Geometry check sheet. Reference: the model listing, model coordinates, mm. A direction names the side the tool comes from. Round coordinates to 2 decimals unless told otherwise and drop trailing zeros. Order: outer loops, then holes, each group sorted by start corner. A loop starts at its lowest first (then second) coordinate and runs counter-clockwise, first axis right, second up.
```python
from build123d import *

# Parameters (mm, degrees)
SKETCH3_W           = 120
SKETCH3_H           = 50
BOSS_EXTRUDE1_DEPTH = 5
SKETCH6_R           = 2
CUT_EXTRUDE1_DEPTH  = 5


with BuildPart() as part:
    # Sketch3 → Boss-Extrude1 (new body)
    with BuildSketch(Plane(origin=(0, 0, 0), x_dir=(1, 0, 0), z_dir=(0, 1, 0))):
        Rectangle(SKETCH3_W, SKETCH3_H)
    extrude(amount=BOSS_EXTRUDE1_DEPTH)

    # Sweep1: sweep along a path in Sketch4
    with BuildLine(Plane.XY) as sweep1_path:
        Line((-50, 5), (-50, 25))
        ThreePointArc((-50, 25), (-47.071067812, 32.071067812), (-40, 35))
        Line((-40, 35), (40, 35))
        ThreePointArc((40, 35), (47.071067812, 32.071067812), (50, 25))
        Line((50, 25), (50, 5))
    # Sketch5 → Sweep1 (sweep)
    with BuildSketch(Plane(origin=(0, 5, 0), x_dir=(1, 0, 0), z_dir=(0, 1, 0))):
        with BuildLine():
            Line((-43.257688432, 6), (-43.257688432, -6))
            ThreePointArc((-43.257688432, -6), (-48.257688432, -11), (-53.257688432, -6))
            Line((-53.257688432, -6), (-53.257688432, 6))
            ThreePointArc((-53.257688432, 6), (-48.257688432, 11), (-43.257688432, 6))
        make_face()
    sweep(path=sweep1_path.line)

    # Sketch6 → Cut-Extrude1 (cut)
    with BuildSketch(Plane(origin=(0, 5, 0), x_dir=(1, 0, 0), z_dir=(0, 1, 0))):
        with Locations(Location((-56, 21, 0), (0, 0, 270))):
            Circle(SKETCH6_R)
        with Locations(Location((-50, 21, 0), (0, 0, 270))):
            Circle(SKETCH6_R)
        with Locations(Location((-50, -21, 0), (0, 0, 90))):
            Circle(SKETCH6_R)
        with Locations(Location((-56, -21, 0), (0, 0, 90))):
            Circle(SKETCH6_R)
        with Locations(Location((56, -21, 0), (0, 0, 270))):
            Circle(SKETCH6_R)
        with Locations(Location((50, -21, 0), (0, 0, 270))):
            Circle(SKETCH6_R)
        with Locations(Location((50, 21, 0), (0, 0, 90))):
            Circle(SKETCH6_R)
        with Locations(Location((56, 21, 0), (0, 0, 90))):
            Circle(SKETCH6_R)
    extrude(amount=-CUT_EXTRUDE1_DEPTH, mode=Mode.SUBTRACT)


solid = part.part
```
(1) Set-up check for faces 4 (the flat face through (53.258, 15, 0)), 5 (the flat face through (-53.258, 15, 0)), 6 (the cylindrical face through (42.278, 27.329, -0.084)), 7 (the cylindrical face through (-48.15, 15.14, -11)), 8 (the cylindrical face through (48.37, 14.86, 11)): record each of +Z, -Z, +X, -X, +Y, -Y from which the full face is reachable in a straight line by a thin tool's end or side.
Returned:
face 4: +Z, -Z, +X, +Y
face 5: +Z, -Z, -X, +Y
face 6: +Z, -Z
face 7: -Z
face 8: +Z
(2) Material ranges on line 1 (X direction, y = 3, z = 21); line 2 (X direction, y = 16, z = 4); line 3 (Y direction, x = 28.5, z = 3), recorded low to high.
Returned:
line 1: x = -60 to -58, -54 to -52, -48 to 48, 52 to 54, 58 to 60
line 2: x = -53.26 to -43.26, 43.26 to 53.26
line 3: y = 0 to 5, 28.26 to 38.26
(3) Sectioned sample at C-C, the plane x = 56. Record the cut outline in (y, z), and give its area (3 significant figures).
Returned:
outline: (0, -25) - (5, -25) - (5, -23) - (0, -23) - close; (0, -19) - (5, -19) - (5, 19) - (0, 19) - close; (0, 23) - (5, 23) - (5, 25) - (0, 25) - close
area: 210 mm2
(4) Sectioned sample at B-B, the plane z = 21. Record the cut outline in (x, y).
Returned:
outline: (-60, 0) - (-58, 0) - (-58, 5) - (-60, 5) - close; (-54, 0) - (-52, 0) - (-52, 5) - (-54, 5) - close; (-48, 0) - (48, 0) - (48, 5) - (-48, 5) - close; (52, 0) - (54, 0) - (54, 5) - (52, 5) - close; (58, 0) - (60, 0) - (60, 5) - (58, 5) - close
(5) Sectioned sample at D-D, the plane x = -35. Record the cut outline in (y, z), and give its area (3 significant figures).
Returned:
outline: (0, -25) - (5, -25) - (5, 25) - (0, 25) - close; (28.26, -6) arc R5 ccw to (38.26, -6) - (38.26, 6) arc R5 ccw to (28.26, 6) - close
area: 449 mm2
(6) Sectioned sample at A-A, the plane y = 15.5. Record the cut outline in (x, z).
Returned:
outline: (-53.26, -6) arc R5 ccw to (-43.26, -6) - (-43.26, 6) arc R5 ccw to (-53.26, 6) - close; (43.26, -6) arc R5 ccw to (53.26, -6) - (53.26, 6) arc R5 ccw to (43.26, 6) - close
(7) Draft check along X on faces 1 (the flat face through (-1, 2, -25)), 2 (the cylindrical face through (-48.37, 15.14, 11)), 3 (the flat face through (60, 2, 0)). Enter one of: released by +X, released by -X, zero draft, split by the parting line, or undercut.
Returned:
face 1: zero draft
face 2: undercut
face 3: released by +X
(8) Depth check by flat-ended pin: P1, Ø2, axis at x = 22.5, z = -17.5, coming from the -Y side; P2, Ø4.5, axis at x = -50, z = -21, coming from the +Y side; P3, Ø13, axis at y = 20, z = -0.5, coming from the -X side; P4, Ø6, axis at y = 12.5, z = 0, coming from the +X side. Enter the tip coordinate at first touch or a pass-through.
Returned:
P1: stops at y = 0
P2: stops at y = 5
P3: stops at x = -53.26
P4: stops at x = 53.26
